Geometry: see drawing. Coordinates: mm, zero at the bounding-box minimum. A direction names the side the tool comes from. Round coordinates to 2 decimals unless told otherwise and drop trailing zeros. Write each loop counter-clockwise with the first axis right and the second up, starting at its lowest first coordinate (ties: lowest second). Pieces come first, ordered by that corner, then holes. Notation, with made-up numbers: M 23,-17 L 36,-17 A33 ccw 36,12 Z; hole C 53.25,-23 d9. An arc over 180 degrees is marked long. Write each question's results on one line, items separated by ' | '. Start each with the question number.
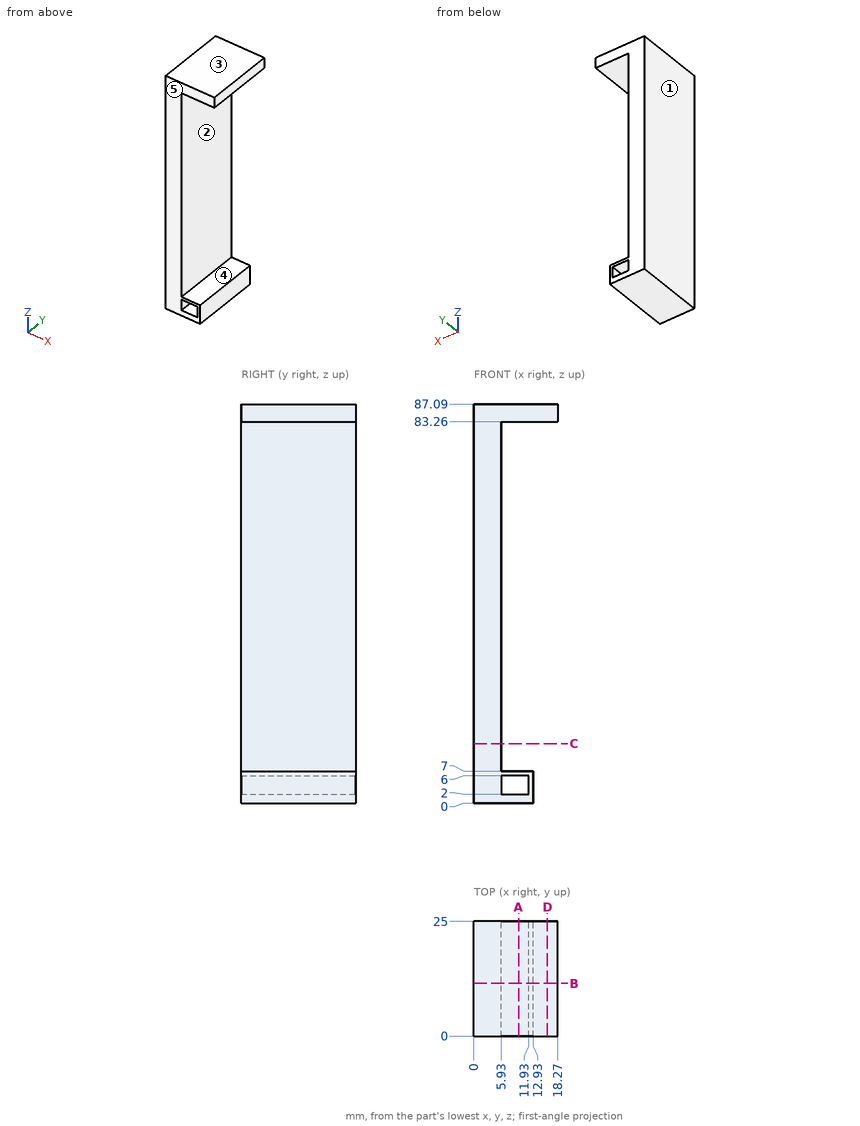
1. Draft query along Z for the marked faces 1, 2 and 3. Return one class per face: +Z half, -Z half, draft (parallel to the pull), parting line (faces both ways), or undercut.
2. Cut plane A-A on x = 9.75. Output: boundary loops of the cut face in (y, z).
3. Contact query for flat-ended pins moving along their axis: P1, Ø10, axis at x = 10.5, y = 17.5, coming from the -Z side; P2, Ø1, axis at y = 19.5, z = 21, coming from the +X side; P3, Ø2, axis at y = 16, z = 4.5, coming from the +X side. Output: stop coordinate, or through.
4. Line query: L1, parallel to Z at x = 6.25, y = 2.75; L2, parallel to Z at x = 12, y = 8; L3, parallel to X at y = 14.5, z = 15. Output: solid intervals per line, ascending. Write a range as from..to.
5. Access query for the marked faces 4 and 5. Directions: +Z, -Z, +X, -X, +Y, -Y. A direction counts if a zero-diameter tool reaches every point of the face in a straight line with its end or side. Return the directions, or none.
6. Cut plane B-B on y = 11.5. Output: boundary loops of the cut face in (x, z), and give its area (3 significant figures).
7. Cut plane D-D on x = 16. Output: boundary loops of the cut face in (y, z).
8. Cut plane C-C on z = 13. Output: boundary loops of the cut face in (x, y), and give its area (3 significant figures).
Answers follow:
1) face 1: draft | face 2: undercut | face 3: +Z half
2) outline: M 0,0 L 25,0 L 25,2 L 0,2 Z; M 0,6 L 25,6 L 25,7 L 0,7 Z; M 0,83.26 L 25,83.26 L 25,87.09 L 0,87.09 Z
3) P1: stops at z = 0 | P2: stops at x = 5.93 | P3: stops at x = 12.93
4) L1: z = 0..2, 6..7, 83.26..87.09 | L2: z = 0..7, 83.26..87.09 | L3: x = 0..5.93
5) face 4: +X, +Y, -Y | face 5: +Z, -Z, +X, -X, -Y
6) outline: M 0,0 L 12.93,0 L 12.93,7 L 5.93,7 L 5.93,83.26 L 18.27,83.26 L 18.27,87.09 L 0,87.09 Z; hole M 5.93,2 L 11.93,2 L 11.93,6 L 5.93,6 Z | area: 589 mm2
7) outline: M 0,83.26 L 25,83.26 L 25,87.09 L 0,87.09 Z
8) outline: M 0,0 L 5.93,0 L 5.93,25 L 0,25 Z | area: 148 mm2
